```python
from build123d import *

# Parameters (mm, degrees)
F0_R     = 5
F0_R_2   = 30
F1_DEPTH = 25


with BuildPart() as f1:
    # F0 (on Front) → F1 (new body, symmetric)
    with BuildSketch(Plane.XZ):
        with BuildLine():
            Line((-60, -10), (-38.729833, -10))
            ThreePointArc((-38.729833, -10), (-36.955181, -15.307337), (-34.457196, -20.31506))
            Line((-34.457196, -20.31506), (-49.497475, -35.355339))
            ThreePointArc((-49.497475, -35.355339), (-49.497475, -49.497475), (-35.355339, -49.497475))
            Line((-35.355339, -49.497475), (-20.31506, -34.457196))
            ThreePointArc((-20.31506, -34.457196), (-5.58247, -39.608535), (10, -38.729833))
            ThreePointArc((10, -38.729833), (15.307337, -36.955181), (20.31506, -34.457196))
            Line((20.31506, -34.457196), (35.355339, -49.497475))
            ThreePointArc((35.355339, -49.497475), (49.497475, -49.497475), (49.497475, -35.355339))
            Line((49.497475, -35.355339), (34.457196, -20.31506))
            ThreePointArc((34.457196, -20.31506), (36.955181, -15.307337), (38.729833, -10))
            Line((38.729833, -10), (60, -10))
            ThreePointArc((60, -10), (70, 0), (60, 10))
            Line((60, 10), (38.729833, 10))
            ThreePointArc((38.729833, 10), (36.955181, 15.307337), (34.457196, 20.31506))
            ThreePointArc((34.457196, 20.31506), (28.284271, 28.284271), (20.31506, 34.457196))
            ThreePointArc((20.31506, 34.457196), (0, 40), (-20.31506, 34.457196))
            Line((-20.31506, 34.457196), (-35.355339, 49.497475))
            ThreePointArc((-35.355339, 49.497475), (-49.497475, 49.497475), (-49.497475, 35.355339))
            Line((-49.497475, 35.355339), (-34.457196, 20.31506))
            ThreePointArc((-34.457196, 20.31506), (-36.955181, 15.307337), (-38.729833, 10))
            Line((-38.729833, 10), (-60, 10))
            ThreePointArc((-60, 10), (-70, 0), (-60, -10))
        make_face()
        with Locations((-42.426407, -42.426407)):
            Circle(F0_R, mode=Mode.SUBTRACT)
        with Locations((-60, 0)):
            Circle(F0_R, mode=Mode.SUBTRACT)
        with Locations((42.426407, -42.426407)):
            Circle(F0_R, mode=Mode.SUBTRACT)
        Circle(F0_R_2, mode=Mode.SUBTRACT)
        with Locations((60, 0)):
            Circle(F0_R, mode=Mode.SUBTRACT)
        with Locations((-42.426407, 42.426407)):
            Circle(F0_R, mode=Mode.SUBTRACT)
        with BuildLine():
            Line((35.355339, 49.497475), (20.31506, 34.457196))
            ThreePointArc((20.31506, 34.457196), (28.284271, 28.284271), (34.457196, 20.31506))
            Line((34.457196, 20.31506), (49.497475, 35.355339))
            ThreePointArc((49.497475, 35.355339), (49.497475, 49.497475), (35.355339, 49.497475))
        make_face()
        with Locations((42.426407, 42.426407)):
            Circle(F0_R, mode=Mode.SUBTRACT)
    extrude(amount=F1_DEPTH, both=True)


solid = f1.part
```
Geometry check sheet. Reference: the model listing, model coordinates, mm. A direction names the side the tool comes from. Give positions to 0.01 mm unless a question says otherwise; leave off trailing zeros. Loops run counter-clockwise (first coordinate to the right, second up) from the corner with the lowest first, then second, coordinate; pieces in that order, holes last. Notation, with made-up numbers: M 55.25,-32.75 L 64.25,-32.75 A20 cw 64.25,-13.75 Z; hole C -29,-28.75 d6. An arc over 180 degrees is marked long. Answer as CSV lines item,"result".
Item 1: Cross-section at A-A on x = 0. Record the cut outline in (y, z).
Values:
outline,"M -25,-40 L 25,-40 L 25,-30 L -25,-30 Z; M -25,30 L 25,30 L 25,40 L -25,40 Z"
Item 2: Cross-section at C-C on y = -0.5. Count the separate pieces of the cut face and the enclosed holes in it, and give its area (3 significant figures).
Values:
separate pieces,"1"
enclosed holes,"7"
area,"5,120 mm²"
Item 3: Access from +Z, -Z, +X, -X, +Y, -Y to the whole of each face (thin tool, end or side, straight path). Record for faces 5 (the flat face through (49, 0, -10)), 6 (the flat face through (27.94, -0.35, 42.08)), 7 (the flat face through (-42.08, -0.35, 27.94)).
Values:
face 5,"+X, +Y, -Y"
face 6,"+Z, +Y, -Y"
face 7,"-X, +Y, -Y"
Item 4: Cross-section at B-B on z = 0. Record the cut outline in (x, y), and give its area (3 significant figures).
Values:
outline,"M -70,-25 L -65,-25 L -65,25 L -70,25 Z; M -55,-25 L -30,-25 L -30,25 L -55,25 Z; M 30,-25 L 55,-25 L 55,25 L 30,25 Z; M 65,-25 L 70,-25 L 70,25 L 65,25 Z"
area,"3,000 mm²"
Item 5: Release check for a two-part mould opening along Z. For faces 1 (the flat face through (41.87, -0.35, 27.73)), 2 (the flat face through (-27.73, -0.35, 41.87)), 3 (the cylindrical face through (49.65, -0.35, 49.34)), 4 (the cylindrical face through (15.2, -0.4, -37)) record: pulls with the +Z half, pulls with the -Z half, needs draft (parallel to the pull), parting line crosses it, or undercut.
Values:
face 1,"undercut"
face 2,"pulls with the +Z half"
face 3,"undercut"
face 4,"pulls with the -Z half"
Item 6: Cross-section at D-D on z = 13. Record the cut outline in (x, y).
Values:
outline,"M -37.83,-25 L -27.04,-25 L -27.04,25 L -37.83,25 Z; M 27.04,-25 L 37.83,-25 L 37.83,25 L 27.04,25 Z"
Item 7: Material ranges on line 1 (Z direction, x = -60, y = 1); line 2 (Z direction, x = 35, y = 10); line 3 (X direction, y = 15.5, z = 42), recorded low to high.
Values:
line 1,"z = -10 to -5, 5 to 10"
line 2,"z = -49.14 to -20.86, -19.36 to 19.36, 20.86 to 49.14"
line 3,"x = -52.42 to -47.41, -37.44 to -27.86, 27.86 to 37.44, 47.41 to 52.42"
Item 8: Depth check by flat-ended pin: P1, Ø5, axis at y = -3.5, z = -15, coming from the +X side; P2, Ø1.5, axis at x = -40.5, y = 5, coming from the +Z side; P3, Ø17, axis at x = -53, y = -7.5, coming from the +Z side; P4, Ø9, axis at x = 60, z = 0, coming from the -Y side. Enter the tip coordinate at first touch or a pass-through.
Values:
P1,"stops at x = 38"
P2,"stops at z = 52.36"
P3,"stops at z = 52.21"
P4,"passes through"
